For this review, take the finished solid that the model builds, in its own axes (mm). Face numbers are marked on the shaded views. A direction names the side the tool comes from. Round coordinates to 2 decimals unless told otherwise and drop trailing zeros. Loops run counter-clockwise (first coordinate to the right, second up) from the corner with the lowest first, then second, coordinate; pieces in that order, holes last.
1) Tool access review of the marked faces 1, 2, 3, 4 and 5: name each direction out of +Z, -Z, +X, -X, +Y, -Y from which nothing blocks a thin tool from reaching the whole face with its end or side.
2) Take a section at A-A (y = 7). State the section outline as (x, z) points.
3) Insertion check: pin 1 (4 mm diameter, centred on x = 0, y = 9, fed in from +Z); pin 2 (1.5 mm diameter, centred on x = -12.5, z = 18.5, fed in from -Y); pin 3 (8.5 mm diameter, centred on y = 8.5, z = -1, fed in from +X). Each pin has a flat end and moves straight along its axis. Give the tip position at first contact, or say it passes through.
4) Take a section at B-B (y = 1.25). State the section outline as (x, z) points.
5) Wall thickness on L1, parallel to Z at x = 0.5, y = 7; L2, parallel to Y at x = -18, z = -22.5; L3, parallel to Y at x = 3.5, z = -15.5: over which ranges is each line inside the solid? List them lowest first.
```python
from build123d import *

# Parameters (mm, degrees)
F0_W     = 50.8
F0_H     = 50.8
F1_DEPTH = 5.08
F2_W     = 9.525
F2_H     = 9.525
F2_W_2   = 3.048
F2_H_2   = 3.048
F3_DEPTH = 12.7
F4_R     = 5.08
F5_R     = 5.08
F6_R     = 24.13
F7_DEPTH = 0.508


# Not quite as in the source:
# - a fillet or chamfer that OpenCascade refuses, or shapes differently, is made with other operations: its cross-section is extruded or revolved along the edge and cut away or added


with BuildPart() as f1:
    # F0 (on Front) → F1 (new body)
    with BuildSketch(Plane.XZ):
        Rectangle(F0_W, F0_H)
    extrude(amount=F1_DEPTH)

    # F2 (on face) → F3 (join)
    with BuildSketch(Plane(origin=(0, 0, 0), x_dir=(-1, 0, 0), z_dir=(0, 1, 0))):
        Rectangle(F2_W, F2_H)
        Rectangle(F2_W_2, F2_H_2, mode=Mode.SUBTRACT)
    extrude(amount=F3_DEPTH)

    # F4
    f4_edges = [f1.edges().sort_by_distance(p)[0] for p in [
        (0, 0, -4.7625),
        (-4.7625, 0, 0),
        (4.7625, 0, 0),
        (0, 0, 4.7625),
    ]]
    fillet(f4_edges, radius=F4_R)

    # F5
    f5_edges = [f1.edges().sort_by_distance(p)[0] for p in [
        (-25.4, -2.54, 25.4),
        (-25.4, -2.54, -25.4),
        (25.4, -2.54, 25.4),
        (25.4, -2.54, -25.4),
    ]]
    fillet(f5_edges, radius=F5_R)

    # F6 (on face) → F7 (cut)
    with BuildSketch(Plane.XZ.offset(5.08)):
        Circle(F6_R)
    extrude(amount=-F7_DEPTH, mode=Mode.SUBTRACT)

    # F8: fillet of radius 457.2 on 1 edges, made by hand

    # F8_s1 → F8_t2 (revolve)
    with BuildSketch(Plane.XY):
        with BuildLine():
            ThreePointArc((24.13, -5.08), (13.3596803239, -4.6990176438), (2.5833729786, -4.572))
            Line((2.5833729786, -4.572), (24.13, -4.572))
            Line((24.13, -4.572), (24.13, -5.08))
        make_face()
    revolve(axis=Axis((0, -4.572, 0), (0, -1, 0)))


solid = f1.part
```
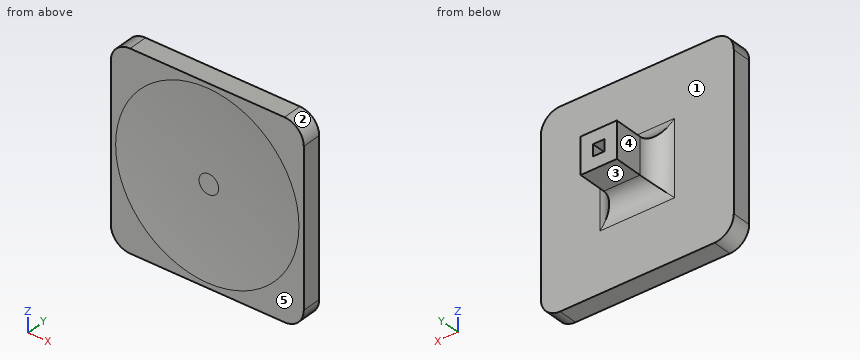
Response:
1. face 1: +Y
1. face 2: +Z, +X, +Y, -Y
1. face 3: -Z, +X, -X, +Y
1. face 4: +Z, -Z, -X, +Y
1. face 5: +Z, -Z, +X, -X, -Y
2. outline: (-4.76, -4.76) - (4.76, -4.76) - (4.76, 4.76) - (-4.76, 4.76) - close; hole (-1.52, -1.52) - (1.52, -1.52) - (1.52, 1.52) - (-1.52, 1.52) - close
3. pin 1: stops at z = 4.76
3. pin 2: stops at y = -5.03
3. pin 3: stops at x = 4.83
4. outline: (-6.51, -6.51) - (6.51, -6.51) - (6.51, 6.51) - (-6.51, 6.51) - close; hole (-1.52, -1.52) - (1.52, -1.52) - (1.52, 1.52) - (-1.52, 1.52) - close
5. L1: z = -4.76 to -1.52, 1.52 to 4.76
5. L2: y = -5.08 to 0
5. L3: y = -4.77 to 0
